The drawing under review shows one solid part. Ordinate dimensions are in mm from its lowest x, y, z. A direction names the side the tool comes from. Coordinates: 2 decimals unless noted, no trailing zeros. Loops run counter-clockwise (first coordinate to the right, second up) from the corner with the lowest first, then second, coordinate; pieces in that order, holes last. Notation, with made-up numbers: M 36.5,85.5 L 44.5,85.5 A21 cw 44.5,116.5 Z; hole C -36,34.25 d8. An arc over 180 degrees is marked long. Put each result on its own line as item: value.
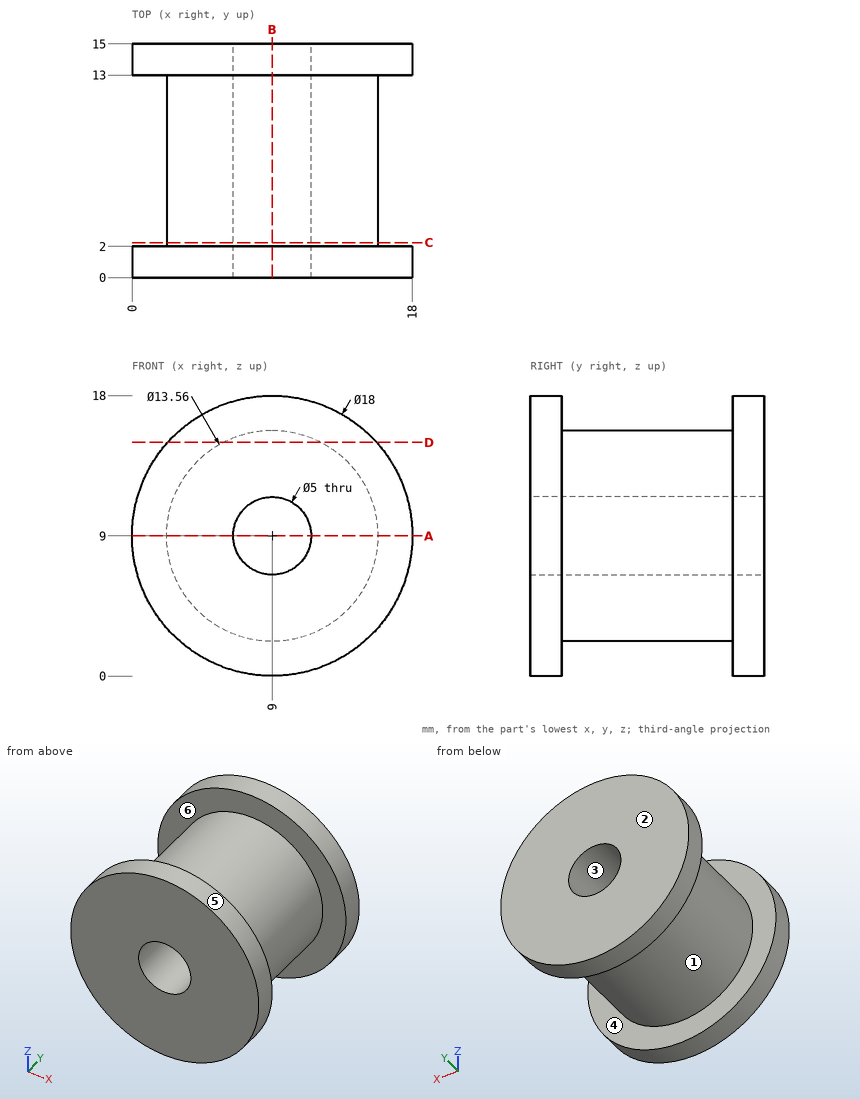
(1) Add section A-A (z = 9). Write out the cut boundary in (x, y), plus the area to 3 significant figures.
Determined:
outline: M 0,0 L 6.5,0 L 6.5,15 L 0,15 L 0,13 L 2.22,13 L 2.22,2 L 0,2 Z; M 11.5,0 L 18,0 L 18,2 L 15.78,2 L 15.78,13 L 18,13 L 18,15 L 11.5,15 Z
area: 146 mm^2
(2) Tool access review of the marked faces 5 and 6: name each direction out of +Z, -Z, +X, -X, +Y, -Y from which nothing blocks a thin tool from reaching the whole face with its end or side.
Determined:
face 5: +Y, -Y
face 6: none
(3) Draft analysis for pull direction Y (two halves, no side actions). For the marked faces 1, 2, 3 and 4, state which applies: +Y half, -Y half, draft (parallel to the pull), parting line (faces both ways), or undercut.
Determined:
face 1: undercut
face 2: +Y half
face 3: draft
face 4: undercut
(4) Add section D-D (z = 15). Write out the cut boundary in (x, y).
Determined:
outline: M 2.29,0 L 15.71,0 L 15.71,2 L 12.16,2 L 12.16,13 L 15.71,13 L 15.71,15 L 2.29,15 L 2.29,13 L 5.84,13 L 5.84,2 L 2.29,2 Z
(5) Add section C-C (y = 2.25). Write out the cut boundary in (x, z), plus the area to 3 significant figures.
Determined:
outline: C 9,9 d13.56; hole C 9,9 d5
area: 125 mm^2
(6) Add section B-B (x = 9). Write out the cut boundary in (y, z).
Determined:
outline: M 0,0 L 2,0 L 2,2.22 L 13,2.22 L 13,0 L 15,0 L 15,6.5 L 0,6.5 Z; M 0,11.5 L 15,11.5 L 15,18 L 13,18 L 13,15.78 L 2,15.78 L 2,18 L 0,18 Z
(7) For pin 1 (1 mm diameter, centred on x = 9.5, y = 10.5, fed in from -Z); pin 2 (1.5 mm diameter, centred on y = 3, z = 8, fed in from +X); pin 3 (3 mm diameter, centred on x = 6.5, y = 9.5, fed in from -Z), all flat-tipped, find the tip position at first contact; note any pin that passes through.
Determined:
pin 1: stops at z = 2.22
pin 2: stops at x = 15.78
pin 3: stops at z = 2.29
(8) Wall thickness on line 1 along X through (y, z) = (5.25, 9); line 2 along Y through (x, z) = (2.25, 11.75); line 3 along Z through (x, y) = (9.5, 6.75): over which ranges is each line inside the solid? List them lowest first. Write a range as [from, to].
Determined:
line 1: x = [2.22, 6.5], [11.5, 15.78]
line 2: y = [0, 2], [13, 15]
line 3: z = [2.24, 6.55], [11.45, 15.76]
